Geometry: final body of the model. Coordinates: model frame, mm. A direction names the side the tool comes from. Give positions to 0.01 mm unless a question says otherwise; leave off trailing zeros. Write each loop counter-clockwise with the first axis right and the second up, starting at its lowest first coordinate (ties: lowest second). Pieces come first, ordered by that corner, then holes. Notation, with made-up numbers: (-26.5, 69) - (-8.5, 69) arc R17 cw to (-8.5, 86) - close; hole circle Ø10 at (56, 68). An arc over 180 degrees is marked (long way). Return JSON: item names as keys, results as strings.
from build123d import *

# Parameters (mm, degrees)
F0_R     = 4.5
F0_R_2   = 4
F1_DEPTH = 1
F0_R_3   = 2.5
F2_DEPTH = 12.9
F3_R     = 0.2
F4_R     = 0.2
F5_R     = 0.2


with BuildPart() as f1:
    # F0 (on Top) → F1 (new body)
    with BuildSketch(Plane.XY):
        Circle(F0_R)
        Circle(F0_R_2, mode=Mode.SUBTRACT)
    extrude(amount=F1_DEPTH)

    # F0 (on Top) → F2 (join)
    with BuildSketch(Plane.XY):
        Circle(F0_R_2)
        Circle(F0_R_3, mode=Mode.SUBTRACT)
    extrude(amount=F2_DEPTH)

    # F3
    f3_edges = [f1.edges().sort_by_distance(p)[0] for p in [
        (-4.5, 0, 0),
    ]]
    fillet(f3_edges, radius=F3_R)

    # F4
    f4_edges = [f1.edges().sort_by_distance(p)[0] for p in [
        (-4.5, 0, 1),
    ]]
    fillet(f4_edges, radius=F4_R)

    # F5
    f5_edges = [f1.edges().sort_by_distance(p)[0] for p in [
        (-4, 0, 12.9),
    ]]
    fillet(f5_edges, radius=F5_R)


solid = f1.part
Q1. Pin query (flat end, axial travel): P1, Ø1, axis at x = 3.5, z = 9.5, coming from the -Y side; P2, Ø1, axis at x = 3.5, z = 3, coming from the +Y side; P3, Ø3, axis at y = 2.5, z = 2, coming from the -X side; P4, Ø3, axis at x = 3, y = -0.5, coming from the -Z side. Return the tip coordinate at first contact, or that it passes through.
Answer key:
{"P1": "stops at y = -2.65", "P2": "stops at y = 2.65", "P3": "stops at x = -4.22", "P4": "stops at z = 0"}
Q2. Material intervals for probe 1 along Y at (x, z) = (0, 5.25); probe 2 along Z at (x, y) = (3.25, 2.75); probe 3 along X at (y, z) = (-1.25, 11.5), sorted ascending. Write a range as [from, to].
Answer key:
{"probe 1": "y = [-4, -2.5], [2.5, 4]", "probe 2": "z = [0, 1]", "probe 3": "x = [-3.8, -2.17], [2.17, 3.8]"}
Q3. Section query A-A, the plane x = 0. Return the cut outline in (y, z), plus the area to 3 significant figures.
Answer key:
{"outline": "(-4.5, 0.2) arc R0.2 ccw to (-4.3, 0) - (-2.5, 0) - (-2.5, 12.9) - (-3.8, 12.9) arc R0.2 ccw to (-4, 12.7) - (-4, 1) - (-4.3, 1) arc R0.2 ccw to (-4.5, 0.8) - close; (2.5, 0) - (4.3, 0) arc R0.2 ccw to (4.5, 0.2) - (4.5, 0.8) arc R0.2 ccw to (4.3, 1) - (4, 1) - (4, 12.7) arc R0.2 ccw to (3.8, 12.9) - (2.5, 12.9) - close", "area": "39.6 mm^2"}
Q4. Section query C-C, the plane z = 7.25. Return the cut outline in (x, y), plus the area to 3 significant figures.
Answer key:
{"outline": "circle Ø8 at (0, 0); hole circle Ø5 at (0, 0)", "area": "30.6 mm^2"}
Q5. Mould query, pull axis X, two halves, no side actions, for faces 1 (the flat face through (2, -2, 0)), 2 (the cylindrical face through (-0.54, -2.44, 6.36)), 3 (the cylindrical face through (-0.59, 4.46, 0.5)). Classes: pulls with the +X half, pulls with the -X half, needs draft (parallel to the pull), parting line crosses it, or undercut.
Answer key:
{"face 1": "needs draft", "face 2": "undercut", "face 3": "parting line crosses it"}
Q6. Set-up query: faces 4 (the cylindrical face through (-0.867, -3.905, 6.768)), 5 (the flat face through (2.5, 0.9, 12.9)). Return all of +Z, -Z, +X, -X, +Y, -Y with unobstructed straight access to the full face (end or side cutting, diameter ignored); none if empty.
Answer key:
{"face 4": "+Z", "face 5": "+Z, +X, -X, +Y, -Y"}
